Design review of the part built by this model. Coordinates are the model's own, in mm. Face numbers are marked on the shaded views. A direction names the side the tool comes from. Coordinates: 2 decimals unless noted, no trailing zeros. Loops run counter-clockwise (first coordinate to the right, second up) from the corner with the lowest first, then second, coordinate; pieces in that order, holes last. Notation, with made-up numbers: (30.5, 4) -> (51.5, 4) arc R7 ccw to (51.5, 13) -> close; hole circle Ø5 at (26.5, 5.5). An arc over 180 degrees is marked (long way). Use CSV: the item, a comma, the result in double quotes.
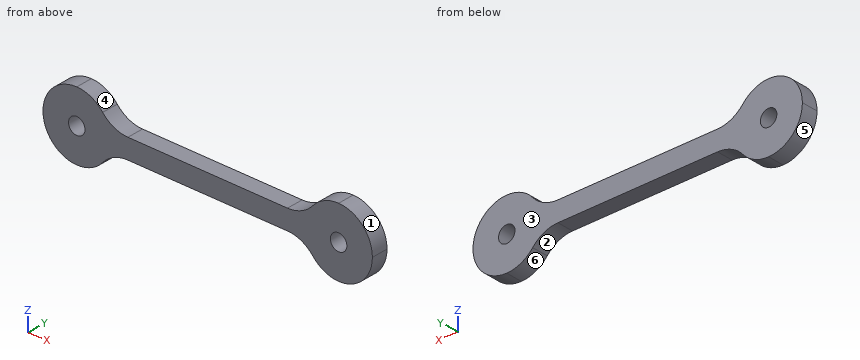
```python
from build123d import *

# Parameters (mm, degrees)
SKETCH1_W           = 100
SKETCH1_H           = 20.5
SKETCH1_R           = 2.5
BOSS_EXTRUDE1_DEPTH = 5
FILLET1_R           = 10.25
CUT_EXTRUDE1_DEPTH  = 10
FILLET2_R           = 10


with BuildPart() as part:
    # Sketch1 → Boss-Extrude1 (new body)
    with BuildSketch(Plane(origin=(0, 0, 0), x_dir=(1, 0, 0), z_dir=(0, 1, 0))):
        with Locations((50, 10.25)):
            Rectangle(SKETCH1_W, SKETCH1_H)
        with Locations(Location((10.25, 10.25, 0), (0, 0, 270))):
            Circle(SKETCH1_R, mode=Mode.SUBTRACT)
        with Locations(Location((89.75, 10.25, 0), (0, 0, 90))):
            Circle(SKETCH1_R, mode=Mode.SUBTRACT)
    extrude(amount=BOSS_EXTRUDE1_DEPTH)

    # Fillet1
    fillet1_edges = [part.edges().sort_by_distance(p)[0] for p in [
        (0, 2.5, 0),
        (0, 2.5, -20.5),
        (100, 2.5, -20.5),
        (100, 2.5, 0),
    ]]
    fillet(fillet1_edges, radius=FILLET1_R - 0.0001)  # a hair under: the kernel refuses the full size

    # Sketch2 → Cut-Extrude1 (cut)
    with BuildSketch(Plane(origin=(0, 5, 0), x_dir=(1, 0, 0), z_dir=(0, 1, 0))):
        with BuildLine():
            Line((20.051147892, 13.25), (79.948852108, 13.25))
            ThreePointArc((79.948852108, 13.25), (83.65440733, 18.490524862), (89.75, 20.5))
            Line((89.75, 20.5), (10.25, 20.5))
            ThreePointArc((10.25, 20.5), (16.34559267, 18.490524862), (20.051147892, 13.25))
        make_face()
        with BuildLine():
            Line((20.051147892, 7.25), (79.948852108, 7.25))
            ThreePointArc((79.948852108, 7.25), (83.65440733, 2.009475138), (89.75, 0))
            Line((89.75, 0), (10.25, 0))
            ThreePointArc((10.25, 0), (16.34559267, 2.009475138), (20.051147892, 7.25))
        make_face()
    extrude(amount=-CUT_EXTRUDE1_DEPTH, mode=Mode.SUBTRACT)

    # Fillet2
    fillet2_edges = [part.edges().sort_by_distance(p)[0] for p in [
        (20.051147892, 2.5, -13.25),
        (79.948852108, 2.5, -13.25),
        (79.948852108, 2.5, -7.25),
        (20.051147892, 2.5, -7.25),
    ]]
    fillet(fillet2_edges, radius=FILLET2_R)


solid = part.part
```
Item 1: Add section C-C (x = 33). Give the boundary of the cut face in (y, z), then the cut area to 3 significant figures.
Checked values:
outline,"(0, -13.25) -> (5, -13.25) -> (5, -7.25) -> (0, -7.25) -> close"
area,"30.0 mm^2"
Item 2: Add section A-A (y = 2.65). State how many separate pieces and enclosed holes the cut face has, then the cut area to 3 significant figures.
Checked values:
separate pieces,"1"
enclosed holes,"2"
area,"994 mm^2"
Item 3: Machinability: for the marked faces 4, 5 and 6, which of the approach directions +Z, -Z, +X, -X, +Y, -Y give a long, thin tool a straight path to every point of the face, cutting with its end or side? Answer none if there is none.
Checked values:
face 4,"+Z, +Y, -Y"
face 5,"-Z, -X, +Y, -Y"
face 6,"-Z, +Y, -Y"
Item 4: Draft analysis for pull direction X (two halves, no side actions). For the marked faces 1, 2 and 3, state which applies: pulls with the +X half, pulls with the -X half, needs draft (parallel to the pull), parting line crosses it, or undercut.
Checked values:
face 1,"pulls with the +X half"
face 2,"undercut"
face 3,"needs draft"
Item 5: Add section D-D (x = 21). Give the boundary of the cut face in (y, z).
Checked values:
outline,"(0, -14.46) -> (5, -14.46) -> (5, -6.04) -> (0, -6.04) -> close"
Item 6: To check wall thickness, follow line 1 along X through (y, z) = (3.15, -10.25); line 2 along X through (y, z) = (0.6, -11.25); line 3 along Z through (x, y) = (89.75, 1.3). State the ranges of each line that lie inside material, in increasing order.
Checked values:
line 1,"0 to 7.75, 12.75 to 87.25, 92.25 to 100"
line 2,"0.05 to 7.96, 12.54 to 87.46, 92.04 to 99.95"
line 3,"-20.5 to -12.75, -7.75 to 0"
Item 7: Add section B-B (z = -4.75). Give the boundary of the cut face in (x, y).
Checked values:
outline,"(1.6, 0) -> (19.16, 0) -> (19.16, 5) -> (1.6, 5) -> close; (80.84, 0) -> (98.4, 0) -> (98.4, 5) -> (80.84, 5) -> close"
Item 8: Clearance check with flat-ended pins moving along their axes: pin 1 (1.5 mm diameter, centred on y = 4, z = -14.5, fed in from +X); pin 2 (2.5 mm diameter, centred on x = 47, y = 2, fed in from -Z); pin 3 (1 mm diameter, centred on y = 0.5, z = -8.5, fed in from -X); pin 4 (4 mm diameter, centred on x = 89.75, z = -10.25, fed in from +Y). State where each tip first meets the part, or that it passes through.
Checked values:
pin 1,"x = 99.38"
pin 2,"z = -13.25"
pin 3,"x = 0.08"
pin 4,"through"
